Could you check a few things on this drawing? It's one solid part, dimensions in mm from its lowest x, y, z. A direction names the side the tool comes from. Coordinates: 2 decimals unless noted, no trailing zeros. Loops run counter-clockwise (first coordinate to the right, second up) from the corner with the lowest first, then second, coordinate; pieces in that order, holes last. Notation, with made-up numbers: M -11.75,-26.75 L 40.25,-26.75 A20 ccw 40.25,12.25 Z; hole C 61,47.5 d9. An arc over 180 degrees is marked long. Answer as a JSON object with one key per item and string values. Group by question number.
Item 1: Suppose I cut it at A-A (z = 1.5). Write out the boundary of the cut face in (x, y).
Item 2: We'd pull the mould along X, two halves only. Please class the marked faces 1, 2, 3 and 4: +X half, -X half, draft (parallel to the pull), parting line (faces both ways), or undercut.
Item 3: If I drill on line 1 (X direction, y = 3.2, z = 0.3) (3 decimals); line 2 (Z direction, x = 6.5, y = 2.8); line 3 (Z direction, x = 9, y = 4.25), over which ranges is the centre line in solid material (lowest first)?
Item 4: Suppose I cut it at B-B (y = 0.8). Write out the boundary of the cut face in (x, z) (3 decimals).
Item 5: Suppose I cut it at D-D (y = 3.05). Count the separate pieces of the cut face and the enclosed holes in it, then the cut area to 3 significant figures.
Item 6: I'm going to push flat-ended pins straight in: pin 1 Ø3 at (x, y) = (11.5, 3.5) entering from -Z; pin 2 Ø1 at (x, z) = (14.5, 4) entering from -Y; pin 3 Ø0.5 at (x, z) = (7.5, 3.5) entering from +Y. Where does each tip first touch, or does it pass through?
Item 7: Suppose I cut it at C-C (x = 14.25). Write out the boundary of the cut face in (y, z).
Item 8: Which directions (+Z, -Z, +X, -X, +Y, -Y) give clear straight access to the entire face, cutting with the end or side of a thin tool? Please do the marked faces 5, 6, 7 and 8.
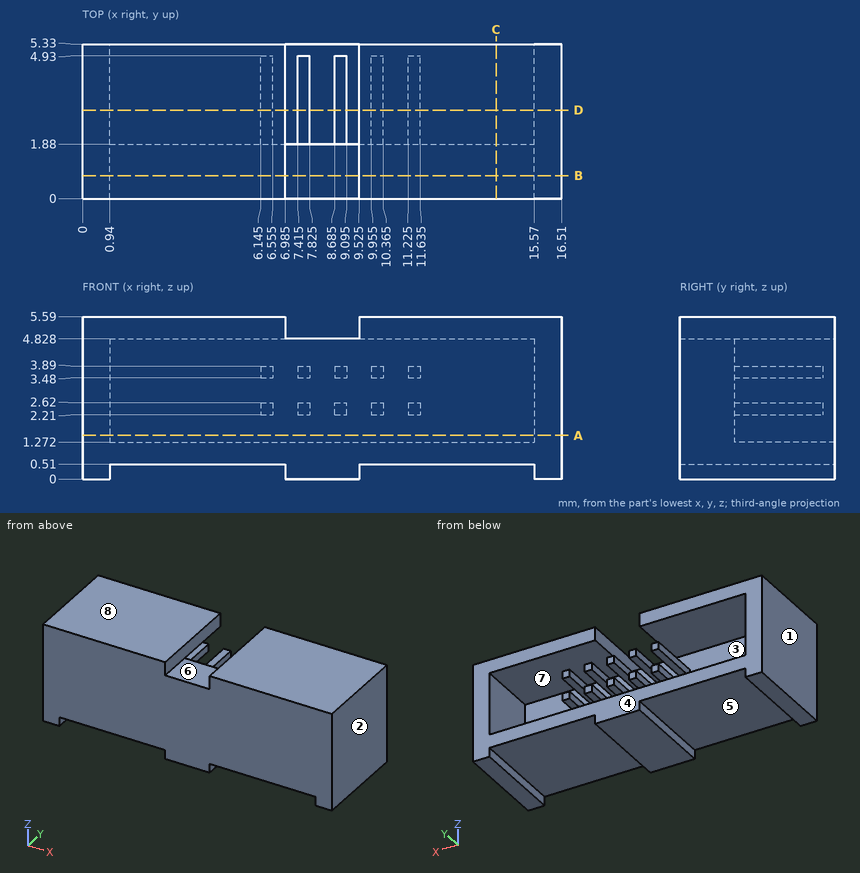
From the geometry:
{
 "1": {"outline": "M 0,0 L 16.51,0 L 16.51,5.33 L 15.57,5.33 L 15.57,1.88 L 0.94,1.88 L 0.94,5.33 L 0,5.33 Z"},
 "2": {"face 1": "-X half", "face 2": "+X half", "face 3": "undercut", "face 4": "draft"},
 "3": {"line 1": "0 to 0.94, 6.985 to 9.525, 15.57 to 16.51", "line 2": "0.51 to 1.27, 2.21 to 2.62, 3.48 to 3.89, 4.83 to 5.59", "line 3": "0 to 1.27, 2.21 to 2.62, 3.48 to 3.89"},
 "4": {"outline": "M 0,0 L 0.94,0 L 0.94,0.51 L 6.985,0.51 L 6.985,0 L 9.525,0 L 9.525,0.51 L 15.57,0.51 L 15.57,0 L 16.51,0 L 16.51,5.59 L 9.525,5.59 L 9.525,4.828 L 6.985,4.828 L 6.985,5.59 L 0,5.59 Z"},
 "5": {"separate pieces": "11", "enclosed holes": "0", "area": "33.8 mm2"},
 "6": {"pin 1": "z = 0.51", "pin 2": "y = 0", "pin 3": "y = 4.93"},
 "7": {"outline": "M 0,0.51 L 5.33,0.51 L 5.33,1.27 L 1.88,1.27 L 1.88,4.83 L 5.33,4.83 L 5.33,5.59 L 0,5.59 Z"},
 "8": {"face 5": "-Z, +Y, -Y", "face 6": "+Z, +Y, -Y", "face 7": "+Y", "face 8": "+Z, +X, -X, +Y, -Y"}
}
